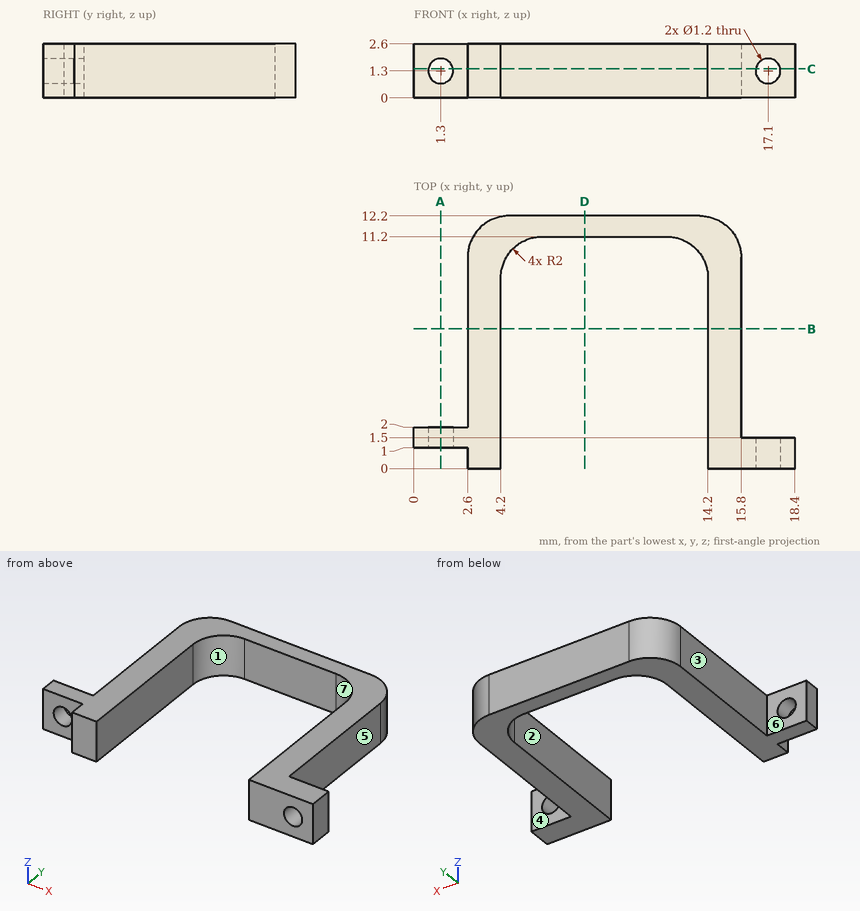
Here's the drawing with two shaded views (mm, measured from the low corner). I have some questions. A direction names the side the tool comes from. Coordinates: 2 decimals unless noted, no trailing zeros. Order: outer loops, then holes, each group sorted by start corner. A loop starts at its lowest first (then second) coordinate and runs counter-clockwise, first axis right, second up. Notation, with made-up numbers: (56.5, -34.5) -> (76.5, -34.5) arc R33 ccw to (76.5, 4.5) -> close; hole circle Ø8 at (18, -5.5). An arc over 180 degrees is marked (long way). One line per question, with ' | ' between items.
Q1. If I drill on L1, parallel to X at y = 1.2, z = 1.3; L2, parallel to X at y = 2.5, z = 1.95; L3, parallel to Y at x = 10.25, z = 1.4, over which ranges is the centre line in solid material (lowest first)?
Return value:
L1: 0 to 0.7, 1.9 to 4.2, 14.2 to 16.5, 17.7 to 18.4 | L2: 2.6 to 4.2, 14.2 to 15.8 | L3: 11.2 to 12.2
Q2. Imagine slicing it at C-C on z = 1.4. Please give me the cut outline in (x, y).
Return value:
outline: (0, 1) -> (0.71, 1) -> (0.71, 2) -> (0, 2) -> close; (1.89, 1) -> (2.6, 1) -> (2.6, 0) -> (4.2, 0) -> (4.2, 9.2) arc R2 cw to (6.2, 11.2) -> (12.2, 11.2) arc R2 cw to (14.2, 9.2) -> (14.2, 0) -> (16.51, 0) -> (16.51, 1.5) -> (15.8, 1.5) -> (15.8, 10.2) arc R2 ccw to (13.8, 12.2) -> (4.6, 12.2) arc R2 ccw to (2.6, 10.2) -> (2.6, 2) -> (1.89, 2) -> close; (17.69, 0) -> (18.4, 0) -> (18.4, 1.5) -> (17.69, 1.5) -> close
Q3. On a 3-axis mill with a long thin cutter (end or side, diameter ignored), from which of +Z, -Z, +X, -X, +Y, -Y can I reach the whole of each face in a straight line? I mean the marked faces 5, 6 and 7. Say none if no direction works.
Return value:
face 5: +Z, -Z, +X, +Y | face 6: +Z, -Z, -X, +Y | face 7: +Z, -Z, -Y
Q4. Imagine slicing it at A-A on x = 1.3. Please give me the cut outline in (y, z).
Return value:
outline: (1, 0) -> (2, 0) -> (2, 0.7) -> (1, 0.7) -> close; (1, 1.9) -> (2, 1.9) -> (2, 2.6) -> (1, 2.6) -> close
Q5. I'm going to push flat-ended pins straight in: P1, Ø1.3, axis at x = 1.5, z = 2, coming from the -Y side; P2, Ø1.4, axis at x = 1.3, z = 1.3, coming from the +Y side; P3, Ø1.3, axis at y = 4, z = 1.5, coming from the -X side. Where does each tip first touch, or does it pass through?
Return value:
P1: y = 1 | P2: y = 2 | P3: x = 2.6
Q6. Thinking about a two-plate mould opening in X: for the marked faces 1, 2, 3 and 4, which applies, pulls with the +X half, pulls with the -X half, needs draft (parallel to the pull), parting line crosses it, or undercut?
Return value:
face 1: undercut | face 2: undercut | face 3: pulls with the -X half | face 4: needs draft
Q7. Imagine slicing it at B-B on y = 6.75. Please give me the cut outline in (x, z), and give its area (3 significant figures).
Return value:
outline: (2.6, 0) -> (4.2, 0) -> (4.2, 2.6) -> (2.6, 2.6) -> close; (14.2, 0) -> (15.8, 0) -> (15.8, 2.6) -> (14.2, 2.6) -> close | area: 8.32 mm²
Q8. Imagine slicing it at D-D on x = 8.25. Please give me the cut outline in (y, z), and give its area (3 significant figures).
Return value:
outline: (11.2, 0) -> (12.2, 0) -> (12.2, 2.6) -> (11.2, 2.6) -> close | area: 2.60 mm²
